```python
from build123d import *

# Parameters (mm, degrees)
F0_R     = 37.592
F1_DEPTH = 4.7625
F3_D     = 16.66748
F4_R     = 2.3622


with BuildPart() as f1:
    # F0 (on Front) → F1 (new body, symmetric)
    with BuildSketch(Plane.XZ):
        Circle(F0_R)
    extrude(amount=F1_DEPTH, both=True)

    # F3 (through all)
    with Locations(Plane.XZ.offset(4.7625)):
        with Locations((0, 0)):
            Hole(F3_D / 2)

    # F4
    f4_edges = [f1.edges().sort_by_distance(p)[0] for p in [
        (-37.592, -4.7625, 0),
        (-37.592, 4.7625, 0),
    ]]
    fillet(f4_edges, radius=F4_R)


solid = f1.part
```
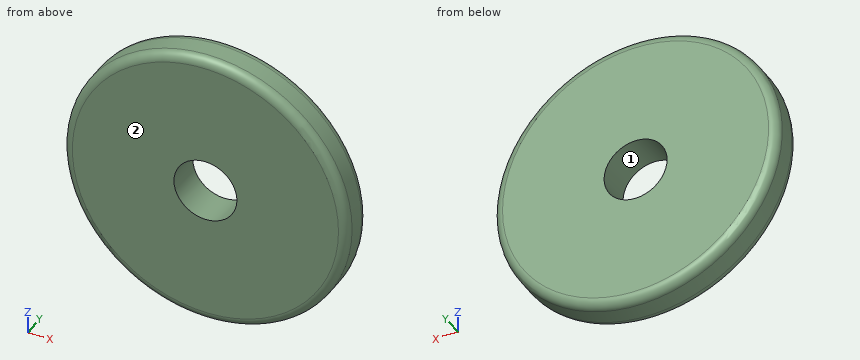
Model file for the job. Use its own axes, mm. Face numbers are marked on the shaded views. Coordinates: 2 decimals unless noted, no trailing zeros. Order: outer loops, then holes, each group sorted by start corner. A loop starts at its lowest first (then second) coordinate and runs counter-clockwise, first axis right, second up. Notation, with made-up numbers: M 17.5,50.5 L 41.5,50.5 A12 ccw 41.5,64.5 Z; hole C 75,54.25 d5. An arc over 180 degrees is marked long. Answer as CSV lines item,"result".
(1) Band-saw the part on A-A, the plane x = 0. List the corners of the cut face in (y, z).
Geometry says:
outline,"M -4.76,-35.23 A2.36 ccw -2.4,-37.59 L 2.4,-37.59 A2.36 ccw 4.76,-35.23 L 4.76,-8.33 L -4.76,-8.33 Z; M -4.76,8.33 L 4.76,8.33 L 4.76,35.23 A2.36 ccw 2.4,37.59 L -2.4,37.59 A2.36 ccw -4.76,35.23 Z"
(2) Band-saw the part on B-B, the plane z = 0. List the corners of the cut face in (x, y).
Geometry says:
outline,"M -37.59,-2.4 A2.36 ccw -35.23,-4.76 L -8.33,-4.76 L -8.33,4.76 L -35.23,4.76 A2.36 ccw -37.59,2.4 Z; M 8.33,-4.76 L 35.23,-4.76 A2.36 ccw 37.59,-2.4 L 37.59,2.4 A2.36 ccw 35.23,4.76 L 8.33,4.76 Z"
(3) Flat gauge pins, fed straight in: pin 1 (15 mm diameter, centred on x = 0, z = 0, fed in from +Y); pin 2 (1 mm diameter, centred on y = -2, z = -19.5, fed in from +X); pin 3 (5 mm diameter, centred on x = 20, y = 3.5, fed in from -Z); pin 4 (1.5 mm diameter, centred on x = 3, y = 2, fed in from +Z). Where does each tip first touch, or does it go through?
Geometry says:
pin 1,"passes through"
pin 2,"stops at x = 32.44"
pin 3,"stops at z = -33.18"
pin 4,"stops at z = 37.52"
(4) Pull direction Z, two halves, no side cores. Call the marked faces 1 and 2: +Z half, -Z half, draft (parallel to the pull), parting line (faces both ways), or undercut.
Geometry says:
face 1,"undercut"
face 2,"draft"
(5) Band-saw the part on C-C, the plane y = 1.25. List the corners of the cut face in (x, z).
Geometry says:
outline,"C 0,0 d75.18; hole C 0,0 d16.67"
(6) Wall check: line 1 along Z through (x, y) = (0, 0.75); line 2 along Z through (x, y) = (0, 3); line 3 along X through (y, z) = (-1, 25). Give the ranges that are in metal, low to high.
Geometry says:
line 1,"z = -37.59 to -8.33, 8.33 to 37.59"
line 2,"z = -37.51 to -8.33, 8.33 to 37.51"
line 3,"x = -28.07 to 28.07"
